Geometry check sheet. Reference: the model listing, model coordinates, mm. Round coordinates to 2 decimals unless told otherwise and drop trailing zeros. Write each loop counter-clockwise with the first axis right and the second up, starting at its lowest first coordinate (ties: lowest second). Pieces come first, ordered by that corner, then holes. Notation, with made-up numbers: M -14.75,23 L 16.25,23 A22 cw 16.25,35 Z; hole C -23.75,36.5 d6. An arc over 180 degrees is marked long. One line per item, written item: value. Start each with the question number.
1. Release check for a two-part mould opening along X. For faces 1 (the flat face through (25, 0, 5)), 2 (the cylindrical face through (24.349, -270.043, 4.93)), 3 (the flat face through (50, -208, 5)) record: pulls with the +X half, pulls with the -X half, needs draft (parallel to the pull), parting line crosses it, or undercut.
2. Scan lines: probe 1 along Y at (x, z) = (25, 8.25); probe 2 along X at (y, z) = (-375, 6.5); probe 3 along X at (y, z) = (-305, 4.25). Record each from-to range of solid material in increasing order. Write a range as [from, to].
3. Section check B-B (z = 6). Record the boundary of the cut face in (x, y), and give its area (3 significant figures).
4. Depth check by flat-ended pin: P1, Ø6, axis at x = 25, y = -275, coming from the -Z side. Enter the tip coordinate at first touch or a pass-through.
5. Section check C-C (y = -375). Record the boundary of the cut face in (x, z), and give its area (3 significant figures).
6. Section check A-A (y = -275). Record the boundary of the cut face in (x, z).
from build123d import *

# Parameters (mm, degrees)
SKETCH1_W           = 50
SKETCH1_H           = 410
SKETCH1_R           = 5
SKETCH1_R_2         = 3
BOSS_EXTRUDE1_DEPTH = 10
FILLET1_R           = 10
SKETCH2_R           = 7.5
CUT_EXTRUDE1_DEPTH  = 10


with BuildPart() as part:
    # Sketch1 → Boss-Extrude1 (new body)
    with BuildSketch(Plane.XY):
        with Locations((25, -205)):
            Rectangle(SKETCH1_W, SKETCH1_H)
        with Locations((25, -275)):
            Circle(SKETCH1_R, mode=Mode.SUBTRACT)
        with Locations((25, -25)):
            Circle(SKETCH1_R, mode=Mode.SUBTRACT)
        with Locations((25, -245)):
            Circle(SKETCH1_R_2, mode=Mode.SUBTRACT)
        with Locations((25, -305)):
            Circle(SKETCH1_R_2, mode=Mode.SUBTRACT)
    extrude(amount=BOSS_EXTRUDE1_DEPTH)

    # Fillet1
    fillet1_edges = [part.edges().sort_by_distance(p)[0] for p in [
        (0, 0, 5),
        (50, 0, 5),
        (50, -410, 5),
        (0, -410, 5),
    ]]
    fillet(fillet1_edges, radius=FILLET1_R)

    # Sketch2 → Cut-Extrude1 (cut)
    with BuildSketch(Plane.XY.offset(10)):
        with Locations((25, -375)):
            Circle(SKETCH2_R)
    extrude(amount=-CUT_EXTRUDE1_DEPTH, mode=Mode.SUBTRACT)


solid = part.part
Result sheet:
1. face 1: needs draft
1. face 2: undercut
1. face 3: pulls with the +X half
2. probe 1: y = [-410, -382.5], [-367.5, -308], [-302, -280], [-270, -248], [-242, -30], [-20, 0]
2. probe 2: x = [0, 17.5], [32.5, 50]
2. probe 3: x = [0, 22], [28, 50]
3. outline: M 0,-400 A10 ccw 10,-410 L 40,-410 A10 ccw 50,-400 L 50,-10 A10 ccw 40,0 L 10,0 A10 ccw 0,-10 Z; hole C 25,-375 d15; hole C 25,-275 d10; hole C 25,-25 d10; hole C 25,-305 d6; hole C 25,-245 d6
3. area: 20,000 mm2
4. P1: passes through
5. outline: M 0,0 L 17.5,0 L 17.5,10 L 0,10 Z; M 32.5,0 L 50,0 L 50,10 L 32.5,10 Z
5. area: 350 mm2
6. outline: M 0,0 L 20,0 L 20,10 L 0,10 Z; M 30,0 L 50,0 L 50,10 L 30,10 Z
